```python
from build123d import *

# Parameters (mm, degrees)
SKIZZE1_W                                   = 130
SKIZZE1_H                                   = 55
AUFSATZ_LINEAR_AUSTRAGEN1_DEPTH             = 10
VERRUNDUNG1_R                               = 10
DURCHGANGSLOCH_F_R_M41_D                    = 4.5
SKIZZE3_R                                   = 11.625
SCHNITT_LINEAR_AUSTRAGEN1_DEPTH             = 5
SKIZZE8_W                                   = 34.5
SKIZZE8_H                                   = 10
SKIZZE8_W_2                                 = 10
SKIZZE8_H_2                                 = 34.5
SCHNITT_LINEAR_AUSTRAGEN3_DEPTH             = 2
SCHNITT_LINEAR_AUSTRAGEN3_DIRECTION_2_REACH = 7
VERRUNDUNG3_R                               = 1.5


with BuildPart() as part:
    # Skizze1 → Aufsatz-Linear austragen1 (new body)
    with BuildSketch(Plane(origin=(0, 0, 0), x_dir=(1, 0, 0), z_dir=(0, 1, 0))):
        with Locations((65, 27.5)):
            Rectangle(SKIZZE1_W, SKIZZE1_H)
    extrude(amount=AUFSATZ_LINEAR_AUSTRAGEN1_DEPTH)

    # Verrundung1
    verrundung1_edges = [part.edges().sort_by_distance(p)[0] for p in [
        (0, 5, -55),
        (130, 5, -55),
        (130, 5, 0),
        (0, 5, 0),
    ]]
    fillet(verrundung1_edges, radius=VERRUNDUNG1_R)

    # Durchgangsloch für M41 (through all)
    with Locations(Plane(origin=(0, 0, 0), x_dir=(-1, 0, 0), z_dir=(0, -1, 0))):
        with Locations((-77.25, 27.5), (-52.75, 27.5), (-28.25, 27.5), (-101.75, 27.5)):
            Hole(DURCHGANGSLOCH_F_R_M41_D / 2)

    # Skizze3 → Schnitt-Linear austragen1 (cut)
    with BuildSketch(Plane(origin=(0, 10, 0), x_dir=(1, 0, 0), z_dir=(0, 1, 0))):
        with Locations((16, 15.25)):
            Circle(SKIZZE3_R)
        with Locations((40.5, 15.25)):
            Circle(SKIZZE3_R)
        with Locations((65, 15.25)):
            Circle(SKIZZE3_R)
        with Locations((89.5, 15.25)):
            Circle(SKIZZE3_R)
        with Locations((114, 15.25)):
            Circle(SKIZZE3_R)
        with Locations((40.5, 39.75)):
            Circle(SKIZZE3_R)
        with Locations((65, 39.75)):
            Circle(SKIZZE3_R)
        with Locations((89.5, 39.75)):
            Circle(SKIZZE3_R)
        with Locations((114, 39.75)):
            Circle(SKIZZE3_R)
        with Locations((16, 39.75)):
            Circle(SKIZZE3_R)
    extrude(amount=-SCHNITT_LINEAR_AUSTRAGEN1_DEPTH, mode=Mode.SUBTRACT)

    # Skizze8 → Schnitt-Linear austragen3 (cut)
    with BuildSketch(Plane(origin=(0, 5, 0), x_dir=(1, 0, 0), z_dir=(0, 1, 0))):
        with Locations((101.75, 39.75)):
            Rectangle(SKIZZE8_W, SKIZZE8_H)
        with Locations((101.75, 15.25)):
            Rectangle(SKIZZE8_W, SKIZZE8_H)
        with Locations((52.75, 39.75)):
            Rectangle(SKIZZE8_W, SKIZZE8_H)
        with Locations((52.75, 15.25)):
            Rectangle(SKIZZE8_W, SKIZZE8_H)
        with Locations((16, 27.5)):
            Rectangle(SKIZZE8_W_2, SKIZZE8_H_2)
    extrude(amount=-SCHNITT_LINEAR_AUSTRAGEN3_DEPTH, mode=Mode.SUBTRACT)

    # Skizze8 → Schnitt-Linear austragen3 direction 2 (cut, up to next)
    with BuildSketch(Plane(origin=(0, 5, 0), x_dir=(1, 0, 0), z_dir=(0, 1, 0)), mode=Mode.PRIVATE) as schnitt_linear_austragen3_direction_2_sk1:
        with Locations((101.75, 39.75)):
            Rectangle(SKIZZE8_W, SKIZZE8_H)
    schnitt_linear_austragen3_direction_2_tool1 = extrude(schnitt_linear_austragen3_direction_2_sk1.sketch, amount=SCHNITT_LINEAR_AUSTRAGEN3_DIRECTION_2_REACH, mode=Mode.PRIVATE) & part.part
    add(schnitt_linear_austragen3_direction_2_tool1.solids().sort_by_distance((101.75, 5, -39.75))[0], mode=Mode.SUBTRACT)
    # Skizze8 → Schnitt-Linear austragen3 direction 2 (cut, up to next)
    with BuildSketch(Plane(origin=(0, 5, 0), x_dir=(1, 0, 0), z_dir=(0, 1, 0)), mode=Mode.PRIVATE) as schnitt_linear_austragen3_direction_2_sk2:
        with Locations((101.75, 15.25)):
            Rectangle(SKIZZE8_W, SKIZZE8_H)
    schnitt_linear_austragen3_direction_2_tool2 = extrude(schnitt_linear_austragen3_direction_2_sk2.sketch, amount=SCHNITT_LINEAR_AUSTRAGEN3_DIRECTION_2_REACH, mode=Mode.PRIVATE) & part.part
    add(schnitt_linear_austragen3_direction_2_tool2.solids().sort_by_distance((101.75, 5, -15.25))[0], mode=Mode.SUBTRACT)
    # Skizze8 → Schnitt-Linear austragen3 direction 2 (cut, up to next)
    with BuildSketch(Plane(origin=(0, 5, 0), x_dir=(1, 0, 0), z_dir=(0, 1, 0)), mode=Mode.PRIVATE) as schnitt_linear_austragen3_direction_2_sk3:
        with Locations((52.75, 39.75)):
            Rectangle(SKIZZE8_W, SKIZZE8_H)
    schnitt_linear_austragen3_direction_2_tool3 = extrude(schnitt_linear_austragen3_direction_2_sk3.sketch, amount=SCHNITT_LINEAR_AUSTRAGEN3_DIRECTION_2_REACH, mode=Mode.PRIVATE) & part.part
    add(schnitt_linear_austragen3_direction_2_tool3.solids().sort_by_distance((52.75, 5, -39.75))[0], mode=Mode.SUBTRACT)
    # Skizze8 → Schnitt-Linear austragen3 direction 2 (cut, up to next)
    with BuildSketch(Plane(origin=(0, 5, 0), x_dir=(1, 0, 0), z_dir=(0, 1, 0)), mode=Mode.PRIVATE) as schnitt_linear_austragen3_direction_2_sk4:
        with Locations((52.75, 15.25)):
            Rectangle(SKIZZE8_W, SKIZZE8_H)
    schnitt_linear_austragen3_direction_2_tool4 = extrude(schnitt_linear_austragen3_direction_2_sk4.sketch, amount=SCHNITT_LINEAR_AUSTRAGEN3_DIRECTION_2_REACH, mode=Mode.PRIVATE) & part.part
    add(schnitt_linear_austragen3_direction_2_tool4.solids().sort_by_distance((52.75, 5, -15.25))[0], mode=Mode.SUBTRACT)
    # Skizze8 → Schnitt-Linear austragen3 direction 2 (cut, up to next)
    with BuildSketch(Plane(origin=(0, 5, 0), x_dir=(1, 0, 0), z_dir=(0, 1, 0)), mode=Mode.PRIVATE) as schnitt_linear_austragen3_direction_2_sk5:
        with Locations((16, 27.5)):
            Rectangle(SKIZZE8_W_2, SKIZZE8_H_2)
    schnitt_linear_austragen3_direction_2_tool5 = extrude(schnitt_linear_austragen3_direction_2_sk5.sketch, amount=SCHNITT_LINEAR_AUSTRAGEN3_DIRECTION_2_REACH, mode=Mode.PRIVATE) & part.part
    add(schnitt_linear_austragen3_direction_2_tool5.solids().sort_by_distance((16, 5, -27.5))[0], mode=Mode.SUBTRACT)

    # Verrundung3
    verrundung3_edges = [part.edges().sort_by_distance(p)[0] for p in [
        (21, 4, -44.75),
        (70, 4, -20.25),
        (70, 4, -44.75),
        (119, 4, -44.75),
        (119, 4, -20.25),
        (11, 4, -10.25),
        (35.5, 4, -34.75),
        (84.5, 4, -34.75),
        (84.5, 4, -10.25),
        (35.5, 4, -10.25),
        (21, 4, -10.25),
        (70, 4, -34.75),
        (70, 4, -10.25),
        (119, 4, -34.75),
        (119, 4, -10.25),
        (35.5, 4, -20.25),
        (84.5, 4, -20.25),
        (84.5, 4, -44.75),
        (35.5, 4, -44.75),
        (11, 4, -44.75),
    ]]
    fillet(verrundung3_edges, radius=VERRUNDUNG3_R)


solid = part.part
```
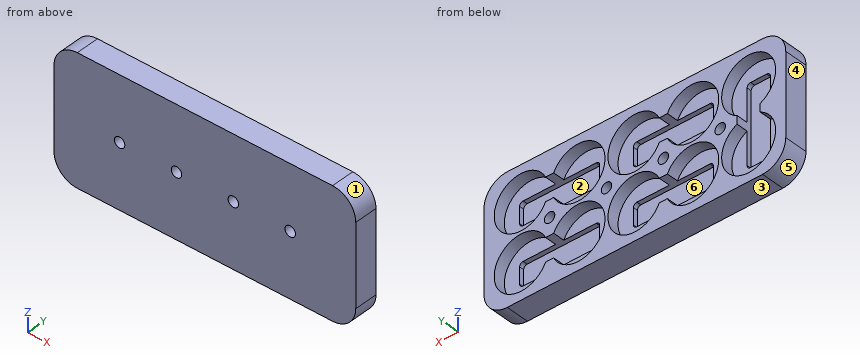
Model file for the job. Use its own axes, mm. Face numbers are marked on the shaded views. A direction names the side the tool comes from. Coordinates: 2 decimals unless noted, no trailing zeros. Loops run counter-clockwise (first coordinate to the right, second up) from the corner with the lowest first, then second, coordinate; pieces in that order, holes last. Notation, with made-up numbers: (47, 25) - (99, 25) arc R14 cw to (99, 38) - close; hole circle Ø1 at (41, 20.5). An arc over 180 degrees is marked (long way). Answer as a JSON object with one key per item and string values. Group by question number.
(1) Probe line 1 along X through (y, z) = (4.75, -39); line 2 along X through (y, z) = (6.75, -27.5); line 3 along Z through (x, y) = (37.5, 4). List the from-to ranges inside material, lowest first.
(2) Two-plate mould, pull along Z, no slides. Class the marked faces 1, 2, 3 and 4: released by +Z, released by -Z, zero draft, split by the parting line, or undercut.
(3) Cut at A-A (x = 52.75). Give the cut face in (y, z).
(4) Cut at B-B (y = 1.75). Give the cut face in (x, z), then the cut area to 3 significant figures.
(5) Cut at C-C (x = 89.5). Give the cut face in (y, z) (3 decimals).
(6) Flat gauge pins, fed straight in: pin 1 (14 mm diameter, centred on x = 40.5, z = -15.25, fed in from +Y); pin 2 (5 mm diameter, centred on x = 107.5, z = -40, fed in from +Y). Where does each tip first touch, or does it go through?
(7) Tool access for the marked faces 5 and 6: list every direction of +Z, -Z, +X, -X, +Y, -Y with a clear straight run to the whole face (end or side of a thin tool).
(8) Cut at D-D (z = -15.25). Give the cut face in (x, y) (3 decimals).
Geometry says:
{
 "1": {"line 1": "x = 0 to 11, 21 to 35.5, 70 to 84.5, 119 to 130", "line 2": "x = 0 to 11, 21 to 26, 30.5 to 50.5, 55 to 75, 79.5 to 99.5, 104 to 130", "line 3": "z = -55 to -44.75, -34.75 to -20.25, -10.25 to 0"},
 "2": {"face 1": "released by +Z", "face 2": "undercut", "face 3": "released by -Z", "face 4": "zero draft"},
 "3": {"outline": "(0, -55) - (10, -55) - (10, -44.75) - (3, -44.75) - (3, -34.75) - (10, -34.75) - (10, -29.75) - (0, -29.75) - close; (0, -25.25) - (10, -25.25) - (10, -20.25) - (3, -20.25) - (3, -10.25) - (10, -10.25) - (10, 0) - (0, 0) - close"},
 "4": {"outline": "(0, -45) arc R10 ccw to (10, -55) - (120, -55) arc R10 ccw to (130, -45) - (130, -10) arc R10 ccw to (120, 0) - (10, 0) arc R10 ccw to (0, -10) - close; hole circle Ø4.5 at (28.25, -27.5); hole circle Ø4.5 at (52.75, -27.5); hole circle Ø4.5 at (77.25, -27.5); hole circle Ø4.5 at (101.75, -27.5)", "area": "7,000 mm^2"},
 "5": {"outline": "(0, -55) - (10, -55) - (10, -51.375) - (5, -51.375) - (5, -44.75) - (3, -44.75) - (3, -34.75) - (5, -34.75) - (5, -28.125) - (10, -28.125) - (10, -26.875) - (5, -26.875) - (5, -20.25) - (3, -20.25) - (3, -10.25) - (5, -10.25) - (5, -3.625) - (10, -3.625) - (10, 0) - (0, 0) - close"},
 "6": {"pin 1": "stops at y = 5", "pin 2": "stops at y = 3"},
 "7": {"face 5": "-Z, -X, +Y, -Y", "face 6": "+Y"},
 "8": {"outline": "(0, 0) - (130, 0) - (130, 10) - (125.625, 10) - (125.625, 5) - (119, 5) - (119, 3) - (84.5, 3) - (84.5, 5) - (77.875, 5) - (77.875, 10) - (76.625, 10) - (76.625, 5) - (70, 5) - (70, 3) - (35.5, 3) - (35.5, 5) - (28.875, 5) - (28.875, 10) - (27.625, 10) - (27.625, 5) - (21, 5) - (21, 3) - (11, 3) - (11, 5) - (4.375, 5) - (4.375, 10) - (0, 10) - close"}
}
